Check sheet for the modelled part. Datum: model origin and axes. Units: mm. Face numbers are marked on the shaded views. A direction names the side the tool comes from. Give positions to 0.01 mm unless a question says otherwise; leave off trailing zeros. Write each loop counter-clockwise with the first axis right and the second up, starting at its lowest first coordinate (ties: lowest second). Pieces come first, ordered by that corner, then holes. Notation, with made-up numbers: (33, 67) -> (67, 67) arc R26 ccw to (67, 93) -> close; hole circle Ø10 at (67, 9). An arc over 180 degrees is marked (long way). Answer as a JSON object with one key per item and string values.
from build123d import *

# Parameters (mm, degrees)
CROSSRECESS_DEPTH = 2.6
FILLET5_R         = 0.3
HEADFILLET_R      = 1
DRAFT1_ANGLE      = 20


with BuildPart() as part:
    # Sketch1 → Base (revolve)
    with BuildSketch(Plane.XY):
        with BuildLine():
            Line((22.6, 2), (4, 2))
            Line((4, 2), (2.9, 2))
            ThreePointArc((2.9, 2), (2.687867966, 2.087867966), (2.6, 2.3))
            Line((2.6, 2.3), (2.6, 3.5))
            Line((2.6, 3.5), (0, 3.272529475))
            Line((0, 3.272529475), (0, 0))
            Line((0, 0), (22.6, 0))
            Line((22.6, 0), (22.6, 2))
        make_face()
    revolve(axis=Axis((4.515812911, 0, 0), (-1, 0, 0)))

    # Sketch6 → CrossRecess (cut)
    with BuildSketch(Plane(origin=(0, 0, 0), x_dir=(0, 0, -1), z_dir=(1, 0, 0))):
        Polygon((0.41, 0.41), (0.41, 2.05), (-0.41, 2.05), (-0.41, 0.41), (-2.05, 0.41), (-2.05, -0.41), (-0.41, -0.41), (-0.41, -2.05), (0.41, -2.05), (0.41, -0.41), (2.05, -0.41), (2.05, 0.41), align=None)
    extrude(amount=CROSSRECESS_DEPTH, mode=Mode.SUBTRACT)

    # Fillet5
    fillet5_edges = [part.edges().sort_by_distance(p)[0] for p in [
        (1.3, 0.41, 0.41),
        (1.3, -0.41, 0.41),
        (1.3, -0.41, -0.41),
        (1.3, 0.41, -0.41),
    ]]
    fillet(fillet5_edges, radius=FILLET5_R)

    # HeadFillet
    headfillet_edges = [part.edges().sort_by_distance(p)[0] for p in [
        (0, -3.272529475, 0),
    ]]
    fillet(headfillet_edges, radius=HEADFILLET_R)

    # Draft1
    draft1_faces = [part.faces().sort_by_distance(p)[0] for p in [
        (1.3, 0, 2.05),
        (1.3, -2.05, 0),
        (1.3, 0, -2.05),
        (1.3, 2.05, 0),
    ]]
    draft(draft1_faces, Plane(origin=(0, 0, 0), x_dir=(0, 0, -1), z_dir=(-1, 0, 0)), DRAFT1_ANGLE)


solid = part.part
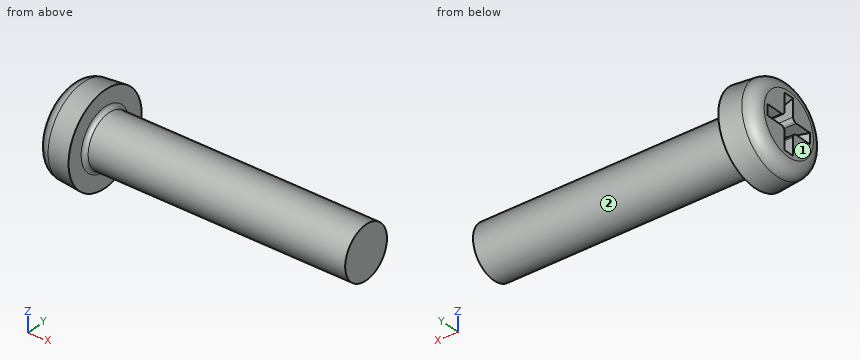
1. Scan lines: L1, parallel to Z at x = 15, y = 0; L2, parallel to Y at x = 7.5, z = 1.75; L3, parallel to X at y = -1, z = 0.25. Record each from-to range of solid material in increasing order. Write a range as [from, to].
Determined:
{"L1": "[-2, 2]", "L2": "[-0.97, 0.97]", "L3": "[2.6, 22.6]"}
2. Go/stop test with flat-tipped pins: P1, Ø0.7, axis at x = 1, z = -1, coming from the -Y side; P2, Ø2, axis at x = 9, y = -2.5, coming from the +Z side; P3, Ø0.7, axis at y = 0, z = 0, coming from the -X side. Record where each tip stops, or that it passes through.
Determined:
{"P1": "y = -3.3", "P2": "z = 1.32", "P3": "x = 2.6"}
3. Sectioned sample at A-A, the plane y = 0. Enter the section's corners in (x, z), plus the area to 3 significant figures.
Determined:
{"outline": "(0, -2.36) arc R1 ccw to (0.91, -3.35) -> (2.6, -3.5) -> (2.6, -2.3) arc R0.3 cw to (2.9, -2) -> (22.6, -2) -> (22.6, 2) -> (2.9, 2) arc R0.3 cw to (2.6, 2.3) -> (2.6, 3.5) -> (0.91, 3.35) arc R1 ccw to (0, 2.36) -> (0, 2.05) -> (2.6, 1.1) -> (2.6, -1.1) -> (0, -2.05) -> close", "area": "89.1 mm^2"}
4. Access from +Z, -Z, +X, -X, +Y, -Y to the whole of each face (thin tool, end or side, straight path). Record for the marked faces 1 and 2.
Determined:
{"face 1": "+Z, -Z, -X, +Y, -Y", "face 2": "+X"}
5. Sectioned sample at C-C, the plane x = 19.25. Enter the section's corners in (y, z), plus the area to 3 significant figures.
Determined:
{"outline": "circle Ø4 at (0, 0)", "area": "12.6 mm^2"}
